Answer from the drawing. Dimensions are ordinates in mm from the lowest x, y and z of the part. A direction names the side the tool comes from. Coordinates: 2 decimals unless noted, no trailing zeros. Write each loop counter-clockwise with the first axis right and the second up, starting at its lowest first coordinate (ties: lowest second). Pieces come first, ordered by that corner, then holes.
(1) The part is cut by section B-B on y = 23.5. Determine the outline of the cut face in (x, z).
(2) The part is cut by section C-C on x = 39. Determine the outline of the cut face in (y, z), plus the area to 3 significant figures.
(3) Which of the six approach directions +Z, -Z, +X, -X, +Y, -Y give full straight-line access (tool end or side, diameter ignored) to the marked faces 4 and 5?
(4) The part is cut by section A-A on z = 36.5. Determine the outline of the cut face in (x, y), plus the area to 3 significant figures.
(5) Straight lines are drawn through the part: line 1 (X direction, y = 22.5, z = 32.5); line 2 (Z direction, x = 9, y = 1); line 3 (Y direction, x = 21, z = 40.5). For each, find the intervals that lie inside material, in ascending order.
(6) Given P1, Ø0.8, axis at x = 53, y = 16.5, coming from the +Z side; P2, Ø8, axis at x = 37.5, z = 17.5, coming from the -Y side; P3, Ø2, axis at x = 52.5, z = 43.5, coming from the -Y side, each flat-ended and moving along its own axis, determine where each tip first touches the part or whether it passes through.
(7) For a pull along X with two mould halves and no side action, classify the marked faces 1, 2 and 3 as +X half, -X half, draft (parallel to the pull), parting line (faces both ways), or undercut.
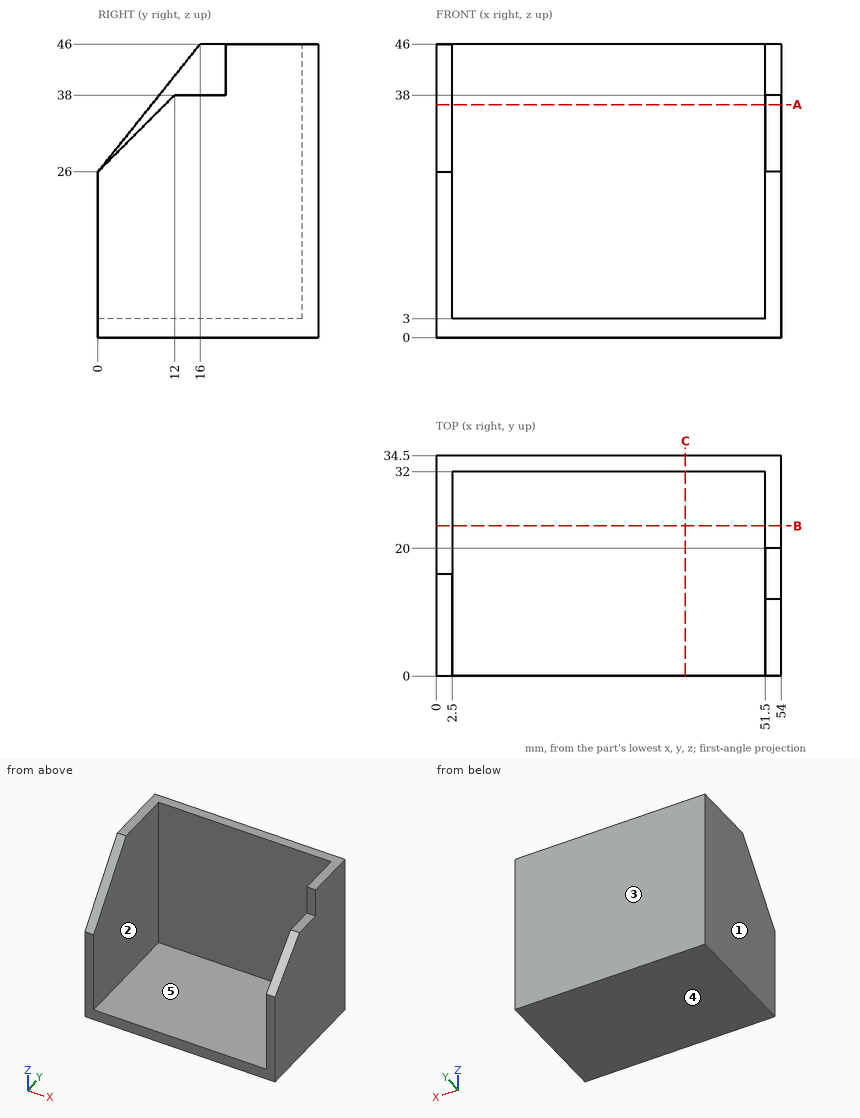
Model answer:
1. outline: (0, 0) - (54, 0) - (54, 46) - (51.5, 46) - (51.5, 3) - (2.5, 3) - (2.5, 46) - (0, 46) - close
2. outline: (0, 0) - (34.5, 0) - (34.5, 46) - (32, 46) - (32, 3) - (0, 3) - close
2. area: 211 mm2
3. face 4: -Z, +X, -X, +Y, -Y
3. face 5: +Z, -Y
4. outline: (0, 8.4) - (2.5, 8.4) - (2.5, 32) - (51.5, 32) - (51.5, 10.5) - (54, 10.5) - (54, 34.5) - (0, 34.5) - close
4. area: 248 mm2
5. line 1: x = 0 to 2.5, 51.5 to 54
5. line 2: z = 0 to 3
5. line 3: y = 32 to 34.5
6. P1: stops at z = 38
6. P2: stops at y = 32
6. P3: stops at y = 20
7. face 1: -X half
7. face 2: undercut
7. face 3: draft
